```python
from build123d import *

# Parameters (mm, degrees)
SKETCH030_R     = 43
SKETCH030_R_2   = 1.765
SKETCH030_R_3   = 1.65
SKETCH030_R_4   = 1.75
PAD005_DEPTH    = 12.5
POCKET001_DEPTH = 10.5
SKETCH032_R     = 3
POCKET002_DEPTH = 3.5


with BuildPart() as part:
    # Sketch030 → Pad005 (new body)
    with BuildSketch(Plane.XY):
        Circle(SKETCH030_R)
        with Locations((-33.5, -16)):
            Circle(SKETCH030_R_2, mode=Mode.SUBTRACT)
        with Locations((17.5, -33)):
            Circle(SKETCH030_R_3, mode=Mode.SUBTRACT)
        with Locations((-11, 36)):
            Circle(SKETCH030_R_4, mode=Mode.SUBTRACT)
    extrude(amount=PAD005_DEPTH)

    # Sketch031 (on Face6 of Pad005) → Pocket001 (cut)
    with BuildSketch(Plane.XY.offset(12.5)):
        with BuildLine():
            Line((11.296867, 36.481132), (53.761138, -10.905243))
            Line((53.761138, -10.905243), (26.20627, -35.59794))
            Line((26.20627, -35.59794), (16.463311, -24.725657))
            Line((16.463311, -24.725657), (26.618554, -15.625256))
            ThreePointArc((26.618554, -15.625256), (26.734588, -13.507112), (24.616444, -13.391078))
            Line((24.616444, -13.391078), (1.902296, -33.745868))
            ThreePointArc((-11.896643, -32.989949), (-5.153729, -36.225762), (1.902296, -33.745868))
            Line((-11.896643, -32.989949), (-36.094334, -5.987464))
            ThreePointArc((-35.338415, 7.811475), (-38.574228, 1.068561), (-36.094334, -5.987464))
            Line((-35.338415, 7.811475), (-2.502071, 37.237051))
            ThreePointArc((11.296867, 36.481132), (4.553954, 39.716945), (-2.502071, 37.237051))
        make_face()
    extrude(amount=-POCKET001_DEPTH, mode=Mode.SUBTRACT)

    # Sketch032 → Pocket002 (cut)
    with BuildSketch(Plane.XY):
        with Locations((-33.5, -16)):
            Circle(SKETCH032_R)
        with Locations((17.5, -33)):
            Circle(SKETCH032_R)
        with Locations((-11, 36)):
            Circle(SKETCH032_R)
    extrude(amount=POCKET002_DEPTH, mode=Mode.SUBTRACT)


with BuildPart() as part_1:
    # Body007 placement: moved
    add(part.part.moved(Location((0, 0, -12.46))))


solid = part_1.part
```
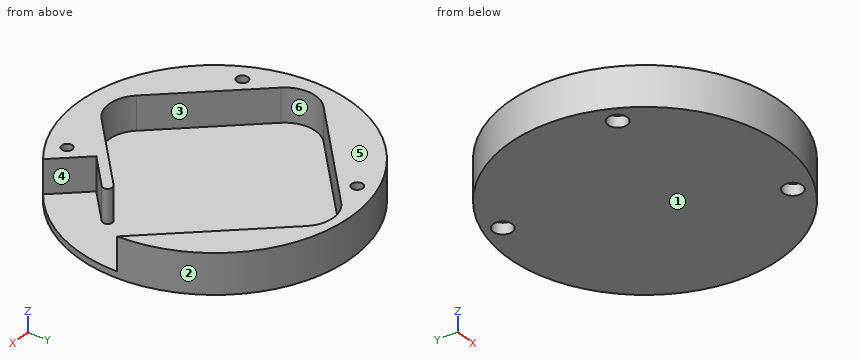
The model under review builds one solid part; all positions refer to its coordinate system, in mm. Face numbers are marked on the shaded views. A direction names the side the tool comes from. Give positions to 0.01 mm unless a question says otherwise; leave off trailing zeros. Write each loop counter-clockwise with the first axis right and the second up, starting at its lowest first coordinate (ties: lowest second). Pieces come first, ordered by that corner, then holes.
(1) Tool access review of the marked faces 5 and 6: name each direction out of +Z, -Z, +X, -X, +Y, -Y from which nothing blocks a thin tool from reaching the whole face with its end or side.
(2) The part is to be moulded in two halves that separate along X. For the marked faces 1, 2, 3 and 4, say which applies: released by +X, released by -X, zero draft, split by the parting line, or undercut.
(3) Consider section A-A, the plane x = -33.5. Give the boundary of the cut face in (y, z) (3 decimals), and give its area (3 significant figures).
(4) To check wall thickness, follow L1, parallel to X at y = -33, z = -4.5; L2, parallel to Y at x = 17.5, z = -9.9; L3, parallel to Y at x = 24.5, z = -3. State the ranges of each line that lie inside material, in increasing order.
(5) Consider section D-D, the plane x = 17.5. Give the boundary of the cut face in (y, z).
(6) For P1, Ø1.5, axis at x = -31, y = -2.5, coming from the +Z side; P2, Ø1, axis at y = 11, z = -6.5, coming from the +X side; P3, Ø7, axis at x = 17.5, y = -33, coming from the +Z side; P4, Ø4.5, axis at x = 17.5, y = -33, coming from the -Z side, all flat-tipped, find the tip position at first contact; note any pin that passes through.
(7) Consider section C-C, the plane y = -27.5. Give the boundary of the cut face in (x, z), and give its area (3 significant figures).
(8) Consider section B-B, the plane z = -3. Give the number of separate pieces and of enclosed holes in the cut face, and give its area (3 significant figures).
Returned:
1. face 5: +Z, +X, -X, +Y, -Y
1. face 6: +Z
2. face 1: zero draft
2. face 2: split by the parting line
2. face 3: undercut
2. face 4: released by +X
3. outline: (-26.958, -12.46) - (-19, -12.46) - (-19, -8.96) - (-17.765, -8.96) - (-17.765, 0.04) - (-26.958, 0.04) - close; (-14.235, -8.96) - (-13, -8.96) - (-13, -12.46) - (26.958, -12.46) - (26.958, 0.04) - (9.459, 0.04) - (9.459, -10.46) - (-8.883, -10.46) - (-8.883, 0.04) - (-14.235, 0.04) - close
3. area: 429 mm2
4. L1: x = -27.57 to -11.89, 2.73 to 15.85, 19.15 to 23.88
4. L2: y = -39.28 to -36, -30 to -25.88, -23.8 to -19.77, 29.56 to 39.28
4. L3: y = -35.34 to -33.69, -17.52 to -13.5, 21.75 to 35.34
5. outline: (-39.28, -12.46) - (-36, -12.46) - (-36, -8.96) - (-34.65, -8.96) - (-34.65, 0.04) - (-39.28, 0.04) - close; (-31.35, -8.96) - (-30, -8.96) - (-30, -12.46) - (39.28, -12.46) - (39.28, 0.04) - (29.56, 0.04) - (29.56, -10.46) - (-19.77, -10.46) - (-19.77, 0.04) - (-23.8, 0.04) - (-23.8, -10.46) - (-25.88, -10.46) - (-25.88, 0.04) - (-31.35, 0.04) - close
6. P1: stops at z = -10.46
6. P2: stops at x = 41.7
6. P3: stops at z = 0.04
6. P4: stops at z = -8.96
7. outline: (-33.06, -12.46) - (33.06, -12.46) - (33.06, -10.46) - (18.95, -10.46) - (18.95, 0.04) - (8.87, 0.04) - (8.87, -10.46) - (-16.82, -10.46) - (-16.82, 0.04) - (-33.06, 0.04) - close
7. area: 409 mm2
8. separate pieces: 1
8. enclosed holes: 3
8. area: 1,870 mm2
